Verification items for the finished model (mm, model axes). Coordinates: 2 decimals unless noted, no trailing zeros. Write each loop counter-clockwise with the first axis right and the second up, starting at its lowest first coordinate (ties: lowest second). Pieces come first, ordered by that corner, then holes. Notation, with made-up numbers: (53, 84) -> (101, 84) arc R6 cw to (101, 90) -> close; hole circle Ø11 at (56.5, -9). An arc over 180 degrees is marked (long way). Write item = value, one per line. Start each with the question number.
(1) Section check B-B (y = 3.5). Record the cut outline in (x, z).
(2) Section check D-D (y = -27). Record the cut outline in (x, z), plus the area to 3 significant figures.
(3) Gauge pin test, flat ends, axial feed: pin 1 Ø3.5 at (y, z) = (-26, 103.5) entering from -X; pin 2 Ø10 at (y, z) = (-18, 70) entering from -X; pin 3 Ø12 at (x, y) = (-75.5, -61) entering from +Z; pin 4 Ø6 at (x, y) = (73, -27) entering from -Z. Record the tip position at first contact, or that the pin passes through.
(4) Section check C-C (z = 33). Record the cut outline in (x, y).
(5) Material ranges on probe 1 along X at (y, z) = (-64.5, 76); probe 2 along Z at (x, y) = (17, -66); probe 3 along X at (y, z) = (-24, 136), recorded low to high. Write a range as [from, to].
(6) Section check A-A (x = -2.5). Record the cut outline in (y, z), plus the area to 3 significant figures.
```python
from build123d import *

# Parameters (mm, degrees)
F0_W     = 254
F0_H     = 101.6
F1_DEPTH = 25.4
F2_W     = 52.7394
F2_H     = 101.6
F3_DEPTH = 127
F5_DEPTH = 25.4
F6_R     = 5.08


with BuildPart() as f1:
    # F0 (on Top) → F1 (new body)
    with BuildSketch(Plane.XY):
        with Locations((5.498968, -27.346462)):
            Rectangle(F0_W, F0_H)
    extrude(amount=F1_DEPTH)

    # F2 (on face) → F3 (join)
    with BuildSketch(Plane.XY.offset(25.4)):
        with Locations((106.129268, -27.346462)):
            Rectangle(F2_W, F2_H)
    extrude(amount=F3_DEPTH)

    # F4 (on face) → F5 (join)
    with BuildSketch(Plane(origin=(79.759568, 0, 0), x_dir=(0, -1, 0), z_dir=(-1, 0, 0))):
        with BuildLine():
            ThreePointArc((31.156462, 137.818299), (27.346462, 138.203187), (23.536462, 137.818299))
            Line((23.536462, 137.818299), (23.536462, 130.198299))
            Line((23.536462, 130.198299), (31.156462, 130.198299))
            Line((31.156462, 130.198299), (31.156462, 137.818299))
        make_face()
        with BuildLine():
            Line((23.642148, 108.086814), (23.642148, 100.466814))
            ThreePointArc((23.642148, 100.466814), (27.346462, 100.103187), (31.050777, 100.466814))
            Line((31.050777, 100.466814), (31.050777, 108.086814))
            Line((31.050777, 108.086814), (23.642148, 108.086814))
        make_face()
    extrude(amount=F5_DEPTH)

    # F6
    f6_edges = [f1.edges().sort_by_distance(p)[0] for p in [
        (-20.870732, -78.146462, 25.4),
        (-121.501032, -27.346462, 25.4),
        (-20.870732, 23.453538, 25.4),
    ]]
    fillet(f6_edges, radius=F6_R)


solid = f1.part
```
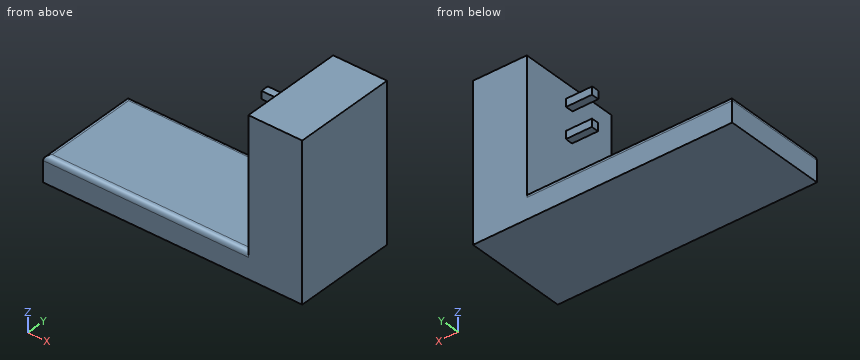
Response:
q1.outline = (-121.5, 0) -> (132.5, 0) -> (132.5, 152.4) -> (79.76, 152.4) -> (79.76, 25.4) -> (-116.42, 25.4) arc R5.08 ccw to (-121.5, 20.32) -> close
q2.outline = (-121.5, 0) -> (132.5, 0) -> (132.5, 152.4) -> (79.76, 152.4) -> (79.76, 138.2) -> (54.36, 138.2) -> (54.36, 130.2) -> (79.76, 130.2) -> (79.76, 108.09) -> (54.36, 108.09) -> (54.36, 100.11) -> (79.76, 100.11) -> (79.76, 25.4) -> (-116.42, 25.4) arc R5.08 ccw to (-121.5, 20.32) -> close
q2.area = 13,500 mm2
q3.pin_1 = 54.36
q3.pin_2 = 79.76
q3.pin_3 = 25.4
q3.pin_4 = 0
q4.outline = (79.76, -78.15) -> (132.5, -78.15) -> (132.5, 23.45) -> (79.76, 23.45) -> close
q5.probe_1 = [79.76, 132.5]
q5.probe_2 = [0, 25.4]
q5.probe_3 = [54.36, 132.5]
q6.outline = (-78.15, 0) -> (23.45, 0) -> (23.45, 20.32) arc R5.08 ccw to (18.37, 25.4) -> (-73.07, 25.4) arc R5.08 ccw to (-78.15, 20.32) -> close
q6.area = 2,570 mm2
